Autodesk Inventor part; units mm, degrees
ref_plane "YZ Plane" through (0, 0, 0) normal (1, 0, 0) x (0, 1, 0)
ref_plane "XZ Plane" through (0, 0, 0) normal (0, 1, 0) x (-1, 0, 0)
ref_plane "XY Plane" through (0, 0, 0) normal (0, 0, 1) x (1, 0, 0)
sketch "Sketch1" plane through (0, 0, 0) normal (0, 0, 1) x (1, 0, 0)
  line L0 (68.7158, -98.8819) -> (-121.2842, -98.8819) construction
  line L1 (-121.2842, -98.8819) -> (-26.2842, 65.663) construction
  line L2 (-26.2842, 65.663) -> (-26.2842, -98.8819) construction
  line L3 (68.7158, -98.8819) -> (-73.7842, -16.6094) construction
  line L4 (-33.7842, -98.8819) -> (-33.7842, -68.8819)
  line L5 (-33.7842, -68.8819) -> (-18.7842, -68.8819)
  line L6 (-18.7842, -68.8819) -> (-18.7842, -98.8819)
  line L7 (-70.0342, -10.1143) -> (-44.0535, -25.1143)
  line L8 (-44.0535, -25.1143) -> (-51.5535, -38.1046)
  line L9 (-51.5535, -38.1046) -> (-77.5342, -23.1046)
  line L10 (-77.5342, -23.1046) -> (-121.2842, -98.8819)
  line L11 (-33.7842, -98.8819) -> (-121.2842, -98.8819)
  line L12 (-18.7842, -98.8819) -> (68.7158, -98.8819)
  line L13 (-26.2842, 65.663) -> (-70.0342, -10.1143)
  line L14 (-121.2842, -98.8819) -> (17.4658, -18.7745) construction
  line L15 (-26.2842, 65.663) -> (68.7158, -98.8819) construction
  line L16 (17.4658, -10.1143) -> (-8.515, -25.1143)
  line L17 (-8.515, -25.1143) -> (-1.015, -38.1046)
  line L18 (-1.015, -38.1046) -> (24.9658, -23.1046)
  line L19 (-26.2842, 65.663) -> (17.4658, -10.1143)
  line L20 (24.9658, -23.1046) -> (68.7158, -98.8819)
  point P0 (-26.2842, -44.0336)
  point P1 (-26.2842, -44.0336)
  dimension "d3" = 190
  dimension "d6" = 7.5
  dimension "d7" = 15
  dimension "d8" = 30
  dimension "d9" = 15
  dimension "d10" = 7.5
  dimension "d16" = 30
  dimension "d18" = 15
  dimension "d19" = 7.5
  dimension "d20" = 30
extrude "Extrusion2" add sketch "Sketch1" along normal blind 3
fillet "Fillet1" radius 6.75 1 edges at (17.4658, -10.1143, 1.5)
fillet "Fillet2" radius 4 14 edges at (-8.515, -25.1143, 1.5) (24.9658, -23.1046, 1.5) (-1.015, -38.1046, 1.5) (-33.7842, -98.8819, 1.5) (-33.7842, -68.8819, 1.5) (-18.7842, -98.8819, 1.5) (68.7158, -98.8819, 1.5) (-18.7842, -68.8819, 1.5) (-121.2842, -98.8819, 1.5) (-70.0342, -10.1143, 1.5) (-44.0535, -25.1143, 1.5) (-51.5535, -38.1046, 1.5) (-77.5342, -23.1046, 1.5) (-26.2842, 65.663, 1.5)
sketch "Sketch3" plane through (0, 0, 3) normal (0, 0, 1) x (1, 0, 0)
  line L0 (61.7876, -98.8819) -> (-14.7842, -98.8819)
  line L1 (-7.2842, -91.8819) -> (-4.2842, -91.8819)
  line L2 (-4.2842, -91.8819) -> (-4.2842, -96.8819)
  line L3 (-4.2842, -96.8819) -> (-7.2842, -96.8819)
  line L4 (-7.2842, -96.8819) -> (-7.2842, -91.8819)
  line L5 (-18.7842, -94.8819) -> (-18.7842, -72.8819)
  line L6 (-7.2842, -42.3819) -> (-4.2842, -42.3819)
  line L7 (-4.2842, -42.3819) -> (-4.2842, -47.3819)
  line L8 (-4.2842, -47.3819) -> (-7.2842, -47.3819)
  line L9 (-7.2842, -47.3819) -> (-7.2842, -42.3819)
  line L10 (-74.0701, -25.1046) -> (-55.0176, -36.1046)
  line L11 (-117.8201, -92.8819) -> (-79.5342, -26.5687)
  line L12 (11.6201, -13.4893) -> (-5.0509, -23.1143)
  line L13 (-22.8201, 59.663) -> (14.0908, -4.2686)
  line L14 (-34.3845, -23.3069) -> (-32.8845, -25.905)
  line L15 (-32.8845, -25.905) -> (-37.2146, -28.405)
  line L16 (-37.2146, -28.405) -> (-38.7146, -25.8069)
  line L17 (-38.7146, -25.8069) -> (-34.3845, -23.3069)
  line L18 (8.4837, 1.4431) -> (9.9837, -1.155)
  line L19 (9.9837, -1.155) -> (5.6536, -3.655)
  line L20 (5.6536, -3.655) -> (4.1536, -1.0569)
  line L21 (4.1536, -1.0569) -> (8.4837, 1.4431)
  line L22 (-40.1839, -61.412) -> (-38.6839, -58.8139)
  line L23 (-38.6839, -58.8139) -> (-34.3538, -61.3139)
  line L24 (-34.3538, -61.3139) -> (-35.8538, -63.912)
  line L25 (-35.8538, -63.912) -> (-40.1839, -61.412)
  line L26 (-83.0522, -36.662) -> (-81.5522, -34.0639)
  line L27 (-81.5522, -34.0639) -> (-77.222, -36.5639)
  line L28 (-77.222, -36.5639) -> (-78.722, -39.162)
  line L29 (-78.722, -39.162) -> (-83.0522, -36.662)
  line L30 (22.7158, -67.1319) -> (25.7158, -67.1319)
  line L31 (25.7158, -67.1319) -> (25.7158, -72.1319)
  line L32 (25.7158, -72.1319) -> (22.7158, -72.1319)
  line L33 (22.7158, -72.1319) -> (22.7158, -67.1319)
  line L34 (-49.5535, -34.6405) -> (-46.0535, -28.5784)
  line L35 (-6.515, -28.5784) -> (-3.015, -34.6405)
  line L36 (-30.7805, 9.9508) -> (-32.2805, 12.5489)
  line L37 (-32.2805, 12.5489) -> (-27.9504, 15.0489)
  line L38 (-27.9504, 15.0489) -> (-26.4504, 12.4508)
  line L39 (-26.4504, 12.4508) -> (-30.7805, 9.9508)
  line L40 (-75.118, -72.4197) -> (-76.618, -75.0178)
  line L41 (-76.618, -75.0178) -> (-72.2879, -77.5178)
  line L42 (-72.2879, -77.5178) -> (-70.7879, -74.9197)
  line L43 (-70.7879, -74.9197) -> (-75.118, -72.4197)
  line L44 (-68.0342, -6.6502) -> (-29.7483, 59.663)
  line L45 (-47.5176, -23.1143) -> (-66.5701, -12.1143)
  line L46 (26.9658, -26.5687) -> (65.2517, -92.8819)
  line L47 (-61.1393, 5.2922) -> (-129.5703, -113.2338) construction
  line L48 (-129.5703, -98.8819) -> (82.7932, -98.8819) construction
  line L49 (71.7222, -104.0892) -> (-26.7217, 66.4208) construction
  line L50 (-61.1393, 5.2922) -> (-24.7647, 68.2948) construction
  line L51 (-26.2842, 65.663) -> (-26.2842, -98.8819) construction
  line L52 (68.7158, -98.8819) -> (-73.7842, -16.6094) construction
  line L53 (-121.2842, -98.8819) -> (21.2158, -16.6094) construction
  circle A0 centre (-26.2842, -44.0336) radius 92.5 construction
  circle A1 centre (53.8231, -90.2836) radius 3.175
  circle A2 centre (-106.3916, -90.2836) radius 3.175
  circle A3 centre (-26.2842, 48.4664) radius 3.175
  point P0 (0, 0)
  dimension "d35" = 3
  dimension "d36" = 5
  dimension "d38" = 2
  dimension "d41" = 11.5
  dimension "d42" = 3
  dimension "d43" = 5
  dimension "d44" = 44.5
  dimension "d45" = 3
  dimension "d46" = 5
  dimension "d47" = 3
  dimension "d48" = 5
  dimension "d49" = 44.5
  dimension "d50" = 3
  dimension "d51" = 5
  dimension "d52" = 3
  dimension "d53" = 5
  dimension "d54" = 44.5
  dimension "d55" = 2
  dimension "d56" = 11.5
  dimension "d57" = 11.5
  dimension "d58" = 2
  dimension "d59" = 3
  dimension "d60" = 5
  dimension "d61" = 19.75
  dimension "d62" = 30
  dimension "d63" = 5
  dimension "d64" = 3
  dimension "d65" = 30
  dimension "d66" = 19.75
  dimension "d67" = 3
  dimension "d68" = 5
  dimension "d69" = 19.75
  dimension "d70" = 30
  dimension "d72" = 185
  dimension "d73" = 6.35
  dimension "d74" = 6.35
  dimension "d75" = 6.35
extrude "Extrusion4" cut sketch "Sketch3" against normal blind 3
equation "\"d6\" = 0.5 * d7"
equation "\"d9\" = d7"
equation "\"d10\" = d6"
equation "\"d16\" = d15"
equation "\"d18\" = d7"
equation "\"d19\" = d6"
equation "\"d20\" = d16"
equation "\"d55\" = d38"
equation "\"d56\" = d41"
equation "\"d57\" = d56"
equation "\"d58\" = d38"
equation "\"d61\" = 0.5 * d44 - 0.5 * d60"
equation "\"d65\" = d62"
equation "\"d66\" = d61"
equation "\"d69\" = d61"
equation "\"d70\" = d62"
equation "\"d15\" = d8"
properties part number "base"
CAD build for the part. Positions are in the model's coordinates, mm. A direction names the side the tool comes from. Coordinates: 2 decimals unless noted, no trailing zeros. Order: outer loops, then holes, each group sorted by start corner. A loop starts at its lowest first (then second) coordinate and runs counter-clockwise, first axis right, second up.
(1) Saw through at A-A, the plane y = -81.5. Write the cut outline in (x, z), and give its area (3 significant figures).
Solution:
outline: (-111.25, 0) - (-33.78, 0) - (-33.78, 3) - (-111.25, 3) - close; (-18.78, 0) - (58.68, 0) - (58.68, 3) - (-18.78, 3) - close
area: 465 mm2
(2) Which spindle directions (+Z, -Z, +X, -X, +Y, -Y) get a long thin tool onto all of the face, cutting with end or side? Do faces 1 (the face through (-17.64, -97.68, 1.52)), 2 (the face through (-57.177, -17.537, 1.479)), 3 (the face through (-64.41, -30.68, 1.48)). Say none if no direction does.
Solution:
face 1: +Z, -Z, -Y
face 2: +Z, -Z, -X
face 3: +Z, -Z
(3) Saw through at C-C, the plane x = -86. Write the cut outline in (y, z), and give its area (3 significant figures).
Solution:
outline: (-98.88, 0) - (-37.77, 0) - (-37.77, 3) - (-98.88, 3) - close
area: 183 mm2
(4) Pin check, flat tips, straight feed: pin 1 Ø0.9 at (x, z) = (-5, 1) entering from +Y; pin 2 Ø5 at (x, y) = (-26.28, 48.47) entering from -Z; pin 3 Ø0.9 at (y, z) = (-85.5, 2) entering from -X; pin 4 Ø0.9 at (y, z) = (-94, 2) entering from -X. Stop position of each tip, or through.
Solution:
pin 1: stops at y = 29.58
pin 2: passes through
pin 3: stops at x = -113.82
pin 4: stops at x = -118.33
(5) Mould opens along X. For faces 4 (the face through (-32.58, -70.02, 1.52)), 5 (the face through (-28, -35, 0)), 6 (the face through (3.401, -18.234, 1.479)), 7 (the face through (-34.987, -97.741, 1.521)) say: released by +X, released by -X, zero draft, split by the parting line, or undercut.
Solution:
face 4: undercut
face 5: zero draft
face 6: released by +X
face 7: undercut
(6) Saw through at B-B, the plane y = 22. Write the cut outline in (x, z).
Solution:
outline: (-51.49, 0) - (-1.08, 0) - (-1.08, 3) - (-51.49, 3) - close
(7) Saw through at D-D, the plane z = 1.25. Count the separate pieces of the cut face and the enclosed holes in it, and give its area (3 significant figures).
Solution:
separate pieces: 1
enclosed holes: 12
area: 14,000 mm2
(8) Drill centre lines: L1, parallel to X at y = -29.5, z = 1.3; L2, parallel to Y at x = 8.5, z = 2; L3, parallel to Y at x = -37, z = 0.3. Where is each one in solid material? Low to high.
Solution:
L1: x = -81.23 to -66.46, -46.59 to -5.98, 13.89 to 28.66
L2: y = -98.88 to -32.61, -15.29 to -2.01, 1.41 to 5.41
L3: y = -98.8 to -63.25, -59.79 to -28.28, -24.82 to 47.1
